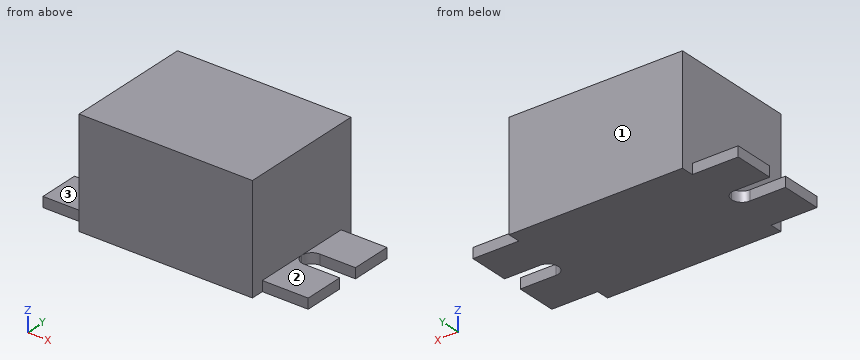
from build123d import *

# Parameters (mm, degrees)
SKETCH1_W           = 34
SKETCH1_H           = 25
BOSS_EXTRUDE1_DEPTH = 21
BOSS_EXTRUDE2_DEPTH = 2


with BuildPart() as part:
    # Sketch1 → Boss-Extrude1 (new body)
    with BuildSketch(Plane.XY):
        with Locations((17, 12.5)):
            Rectangle(SKETCH1_W, SKETCH1_H)
    extrude(amount=BOSS_EXTRUDE1_DEPTH)

    # Sketch3 → Boss-Extrude2 (add)
    with BuildSketch(Plane.XY):
        with BuildLine():
            Line((0, 12.5), (0, 22.5))
            Line((0, 22.5), (-9, 22.5))
            Line((-9, 22.5), (-9, 14.5))
            Line((-9, 14.5), (-2, 14.5))
            ThreePointArc((-2, 14.5), (-0.585786438, 13.914213562), (0, 12.5))
        make_face()
        with BuildLine():
            Line((0, 2.5), (0, 12.5))
            ThreePointArc((0, 12.5), (-0.585786438, 11.085786438), (-2, 10.5))
            Line((-2, 10.5), (-9, 10.5))
            Line((-9, 10.5), (-9, 2.5))
            Line((-9, 2.5), (0, 2.5))
        make_face()
        with BuildLine():
            ThreePointArc((36, 10.5), (34.585786455, 11.08578642), (34, 12.499999949))
            Line((34, 12.499999949), (34, 2.5))
            Line((34, 2.5), (43, 2.5))
            Line((43, 2.5), (43, 10.5))
            Line((43, 10.5), (36, 10.5))
        make_face()
        with BuildLine():
            Line((43, 22.5), (34, 22.5))
            Line((34, 22.5), (34, 12.499999949))
            ThreePointArc((34, 12.499999949), (34.58578642, 13.914213545), (36, 14.5))
            Line((36, 14.5), (43, 14.5))
            Line((43, 14.5), (43, 22.5))
        make_face()
    extrude(amount=BOSS_EXTRUDE2_DEPTH)


solid = part.part
Geometry: final body of the model. Coordinates: model frame, mm. Face numbers are marked on the shaded views. A direction names the side the tool comes from. Coordinates: 2 decimals unless noted, no trailing zeros. Order: outer loops, then holes, each group sorted by start corner. A loop starts at its lowest first (then second) coordinate and runs counter-clockwise, first axis right, second up. Notation, with made-up numbers: M -38,-2.75 L 7,-2.75 A30 cw 7,30.25 Z; hole C 66.5,54.25 d7. An arc over 180 degrees is marked long. One line per question, with ' | ' between items. Start each with the question number.
Item 1: Cut plane D-D, the plane y = 11. Return the cut outline in (x, z).
Item 2: Cut plane A-A, the plane x = 39.5. Return the cut outline in (y, z), then the cut area to 3 significant figures.
Item 3: Set-up query: the marked faces 1, 2 and 3. Return all of +Z, -Z, +X, -X, +Y, -Y with unobstructed straight access to the full face (end or side cutting, diameter ignored); none if empty.
Item 4: Pin query (flat end, axial travel): pin 1 Ø3 at (x, y) = (32, 20) entering from -Z; pin 2 Ø1.6 at (x, z) = (-6, 0.5) entering from +Y; pin 3 Ø1 at (x, z) = (37.5, 1) entering from -Y; pin 4 Ø6.5 at (y, z) = (6.5, 7) entering from -X. Return the tip coordinate at first contact, or that it passes through.
Item 5: Ray query, probe 1 along X at (y, z) = (12.25, 11.25); probe 2 along Z at (x, y) = (37, 5.75). Return the intervals inside material, ascending. Write a range as [from, to].
Item 6: Cut plane C-C, the plane z = 13.5. Return the cut outline in (x, y).
Item 7: Cut plane B-B, the plane y = 21.25. Return the cut outline in (x, z).
A:
1) outline: M -0.68,0 L 34.68,0 L 34.68,2 L 34,2 L 34,21 L 0,21 L 0,2 L -0.68,2 Z
2) outline: M 2.5,0 L 10.5,0 L 10.5,2 L 2.5,2 Z; M 14.5,0 L 22.5,0 L 22.5,2 L 14.5,2 Z | area: 32.0 mm2
3) face 1: +Z, -Z, +X, -X, +Y | face 2: +Z, +X, +Y, -Y | face 3: +Z, -X, +Y, -Y
4) pin 1: stops at z = 0 | pin 2: stops at y = 22.5 | pin 3: stops at y = 2.5 | pin 4: stops at x = 0
5) probe 1: x = [0, 34] | probe 2: z = [0, 2]
6) outline: M 0,0 L 34,0 L 34,25 L 0,25 Z
7) outline: M -9,0 L 43,0 L 43,2 L 34,2 L 34,21 L 0,21 L 0,2 L -9,2 Z
